from build123d import *

# Parameters (mm, degrees)
F1_DEPTH = 30.1625
F2_START = 19.05
F2_DEPTH = 11.1125
F3_START = 19.05
F3_DEPTH = 11.1125
F4_R     = 3.302
F6_DEPTH = 57.1533267105
F7_R     = 6.35
F8_DEPTH = 22.353


with BuildPart() as f1:
    # F0 (on Front) → F1 (new body, symmetric)
    with BuildSketch(Plane.XZ):
        with BuildLine():
            ThreePointArc((-171.8564, 22.352), (-194.2084, 44.704), (-216.5604, 22.352))
            Line((-216.5604, 22.352), (-206.9084, 22.352))
            ThreePointArc((-206.9084, 22.352), (-194.2084, 35.052), (-181.5084, 22.352))
            Line((-181.5084, 22.352), (-171.8564, 22.352))
        make_face()
        with BuildLine():
            ThreePointArc((-216.5604, 22.352), (-210.0136507731, 6.5467492269), (-194.2084, 0))
            ThreePointArc((-194.2084, 0), (-178.4031492269, 6.5467492269), (-171.8564, 22.352))
            Line((-171.8564, 22.352), (-181.5084, 22.352))
            ThreePointArc((-181.5084, 22.352), (-194.2084, 9.652), (-206.9084, 22.352))
            Line((-206.9084, 22.352), (-216.5604, 22.352))
        make_face()
        Polygon((-165.9270077944, 0), (-102.362, 0), (-108.3564, 22.352), (-165.9270077944, 22.352), align=None)
        with BuildLine():
            Line((-76.962, 0), (0, 0))
            Line((0, 0), (0, 14.478))
            ThreePointArc((0, 14.478), (-2.3062412049, 20.0457587951), (-7.874, 22.352))
            Line((-7.874, 22.352), (-44.1198, 22.352))
            Line((-44.1198, 22.352), (-76.962, 22.352))
            Line((-76.962, 22.352), (-76.962, 0))
        make_face()
        Polygon((-102.362, 0), (-76.962, 0), (-76.962, 22.352), (-108.3564, 22.352), align=None)
        with BuildLine():
            Line((-194.2084, 0), (-165.9270077944, 0))
            Line((-165.9270077944, 0), (-165.9270077944, 22.352))
            Line((-165.9270077944, 22.352), (-171.8564, 22.352))
            ThreePointArc((-171.8564, 22.352), (-178.4031492269, 6.5467492269), (-194.2084, 0))
        make_face()
    extrude(amount=F1_DEPTH, both=True)

    # F0 (on Front) → F2 (join)
    with BuildSketch(Plane.XZ.offset(F2_START)):
        with BuildLine():
            ThreePointArc((-63.1698, 57.1523267105), (-66.7435560249, 38.4354391488), (-76.962, 22.352))
            Line((-76.962, 22.352), (-44.1198, 22.352))
            Line((-44.1198, 22.352), (-44.1198, 52.0723267105))
            ThreePointArc((-44.1198, 52.0723267105), (-45.6076975516, 55.664429159), (-49.1998, 57.1523267105))
            Line((-49.1998, 57.1523267105), (-63.1698, 57.1523267105))
        make_face()
    extrude(amount=F2_DEPTH)

    # F0 (on Front) → F3 (cut)
    with BuildSketch(Plane.XZ.offset(F3_START)):
        Polygon((-102.362, 0), (-76.962, 0), (-76.962, 22.352), (-108.3564, 22.352), align=None)
    extrude(amount=F3_DEPTH, mode=Mode.SUBTRACT)

    # F4
    f4_edges = [f1.edges().sort_by_distance(p)[0] for p in [
        (-171.8564, 0, 22.352),
    ]]
    fillet(f4_edges, radius=F4_R)

    # F5 (on Top) → F6 (cut, through all)
    with BuildSketch(Plane.XY):
        Polygon((-165.4523751593, -11.1633), (-165.4523751593, 0), (-165.4523751593, 11.1633), (-218.2923191004, 11.1633), (-218.2923191004, -11.1633), align=None)
    extrude(amount=F6_DEPTH, mode=Mode.SUBTRACT)

    # F7 (on face) → F8 (cut, through all)
    with BuildSketch(Plane.XY.offset(22.352)):
        with Locations((-38.862, 7.8105)):
            Circle(F7_R)
    extrude(amount=-F8_DEPTH, mode=Mode.SUBTRACT)


solid = f1.part
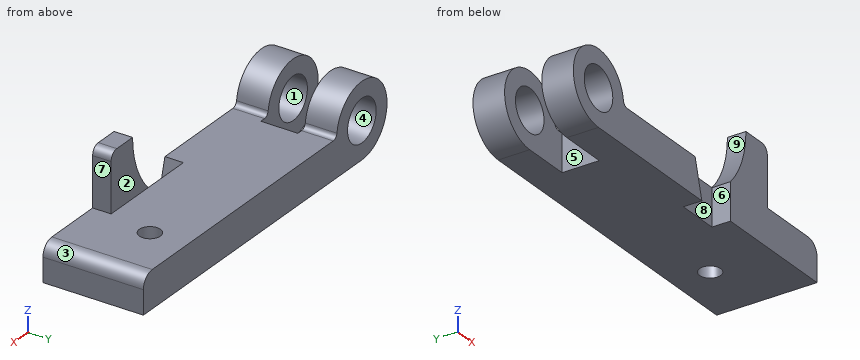
Here's how the part is built. I have some questions about the finished solid (model axes, mm). Face numbers are marked on the shaded views. A direction names the side the tool comes from. Coordinates: 2 decimals unless noted, no trailing zeros. Order: outer loops, then holes, each group sorted by start corner. A loop starts at its lowest first (then second) coordinate and runs counter-clockwise, first axis right, second up. Notation, with made-up numbers: M 31.25,19 L 52.25,19 A29 ccw 52.25,57 Z; hole C -33.75,-3 d6. An arc over 180 degrees is marked long. Answer as CSV lines item,"result". Start each with the question number.
1. I want a section at A-A, the plane y = 21. Write out the boundary of the cut face in (x, z).
2. I want a section at C-C, the plane x = -35. Write out the boundary of the cut face in (y, z), and give its area (3 significant figures).
3. We'd pull the mould along Z, two halves only. Please class the marked faces 1, 2, 3 and 4: released by +Z, released by -Z, zero draft, split by the parting line, or undercut.
4. For pin 1 (13.5 mm diameter, centred on x = -202.5, z = 15.5, fed in from +Y); pin 2 (3 mm diameter, centred on x = -154.5, y = -7.5, fed in from +Z); pin 3 (12 mm diameter, centred on y = -27, z = 13.5, fed in from -X); pin 4 (15 mm diameter, centred on x = -194.21, z = 22.35, fed in from +Y), each with a flat end and sliding along its axis, tell me the tip position at first contact or that it passes through.
5. I need wall thicknesses on line 1 (Y direction, x = -180.5, z = 14.5); line 2 (Z direction, x = -87, y = 8); line 3 (X direction, y = -23.5, z = 17.5). Which ranges of each line are inside material? Lowest first, please. Write a range as [from, to].
6. I want a section at B-B, the plane z = 17.5. Write out the boundary of the cut face in (x, y).
7. I want a section at D-D, the plane z = 30. Write out the boundary of the cut face in (x, y).
8. On a 3-axis mill with a long thin cutter (end or side, diameter ignored), from which of +Z, -Z, +X, -X, +Y, -Y can I reach the whole of each face in a straight line? I mean the marked faces 5, 6, 7, 8 and 9. Say none if no direction works.
Recorded:
1,outline,"M -194.21,0 L 0,0 L 0,14.48 A7.87 ccw -7.87,22.35 L -168.77,22.35 A3.3 cw -172.04,25.23 A22.35 ccw long Z; hole C -194.21,22.35 d25.4"
2,outline,"M -30.16,0 L 2.77,0 L 2.77,22.35 L -30.16,22.35 Z; M 12.85,0 L 30.16,0 L 30.16,22.35 L 12.85,22.35 Z"
2,area,"1,120 mm2"
3,face 1,"undercut"
3,face 2,"zero draft"
3,face 3,"released by +Z"
3,face 4,"undercut"
4,pin 1,"stops at y = 30.16"
4,pin 2,"stops at z = 22.35"
4,pin 3,"stops at x = -216.38"
4,pin 4,"passes through"
5,line 1,"y = [-30.16, -11.16], [11.16, 30.16]"
5,line 2,"z = [0, 22.35]"
5,line 3,"x = [-216.03, -205.95], [-182.47, -107.06], [-76.96, -0.6]"
6,outline,"M -216.03,-30.16 L -205.95,-30.16 L -205.95,-11.16 L -216.03,-11.16 Z; M -216.03,11.16 L -205.95,11.16 L -205.95,30.16 L -216.03,30.16 Z; M -182.47,-30.16 L -107.06,-30.16 L -107.06,-19.05 L -76.96,-19.05 L -76.96,-30.16 L -0.6,-30.16 L -0.6,30.16 L -182.47,30.16 L -182.47,11.16 L -165.45,11.16 L -165.45,-11.16 L -182.47,-11.16 Z; hole C -38.86,7.81 d12.7"
7,outline,"M -215.21,-30.16 L -204.35,-30.16 L -204.35,-11.16 L -215.21,-11.16 Z; M -215.21,11.16 L -204.35,11.16 L -204.35,30.16 L -215.21,30.16 Z; M -184.07,-30.16 L -173.21,-30.16 L -173.21,-11.16 L -184.07,-11.16 Z; M -184.07,11.16 L -173.21,11.16 L -173.21,30.16 L -184.07,30.16 Z; M -71.04,-30.16 L -44.12,-30.16 L -44.12,-19.05 L -71.04,-19.05 Z"
8,face 5,"+Z, -Z, -X"
8,face 6,"+Z, -Z, -Y"
8,face 7,"+Z, +X, +Y, -Y"
8,face 8,"+Z, -Y"
8,face 9,"+Z, +Y, -Y"
